Verification items for the finished model (mm, model axes). Face numbers are marked on the shaded views. A direction names the side the tool comes from. Round coordinates to 2 decimals unless told otherwise and drop trailing zeros. Write each loop counter-clockwise with the first axis right and the second up, starting at its lowest first coordinate (ties: lowest second). Pieces come first, ordered by that corner, then holes. Notation, with made-up numbers: (9, 36) - (40, 36) arc R30 ccw to (40, 65) - close; hole circle Ø3 at (-1.75, 30). An arc over 180 degrees is marked (long way). Answer as a JSON object with one key per item and string values. Group by question number.
1) Thickness scan on line 1 (X direction, y = 4, z = -8); line 2 (X direction, y = 5.5, z = -4); line 3 (X direction, y = 3.75, z = -3.25). Record the ranges inside material, lowest first.
2) Section check B-B (z = 0). Enter the section's corners in (x, y).
3) Set-up check for the marked faces 1, 2 and 3: record each of +Z, -Z, +X, -X, +Y, -Y from which the full face is reachable in a straight line by a thin tool's end or side.
4) Mould release check, pull along X, two halves, no side actions. Record for the marked faces 4, 5 and 6: +X half, -X half, draft (parallel to the pull), parting line (faces both ways), or undercut.
5) Section check D-D (x = 21). Enter the section's corners in (y, z).
6) Go/stop test with flat-tipped pins: pin 1 Ø1.5 at (x, y) = (14, 2) entering from -Z; pin 2 Ø3 at (x, y) = (10, 8) entering from -Z; pin 3 Ø2 at (x, z) = (18, -7) entering from +Y; pin 4 Ø2 at (x, z) = (27.5, -5.5) entering from +Y. Record where each tip stops, or that it passes through.
7) Section check A-A (y = 8). Enter the section's corners in (x, z), then the cut area to 3 significant figures.
```python
from build123d import *

# Parameters (mm, degrees)
F0_R     = 10
F1_DEPTH = 5
F2_R     = 7.5
F3_DEPTH = 5
F4_R     = 10
F5_DEPTH = 5
F6_R     = 5
F7_DEPTH = 20
F8_SIZE  = 1


with BuildPart() as f1:
    # F0 (on Right) → F1 (new body)
    with BuildSketch(Plane.YZ):
        Circle(F0_R)
    extrude(amount=F1_DEPTH)

    # F2 (on face) → F3 (join)
    with BuildSketch(Plane.YZ.offset(5)):
        Circle(F2_R)
    extrude(amount=F3_DEPTH)

    # F4 (on face) → F5 (join)
    with BuildSketch(Plane.YZ.offset(10)):
        Circle(F4_R)
    extrude(amount=F5_DEPTH)

    # F6 (on face) → F7 (join)
    with BuildSketch(Plane.YZ.offset(15)):
        Circle(F6_R)
    extrude(amount=F7_DEPTH)

    # F8
    f8_edges = [f1.edges().sort_by_distance(p)[0] for p in [
        (35, -5, 0),
    ]]
    chamfer(f8_edges, length=F8_SIZE)


solid = f1.part
```
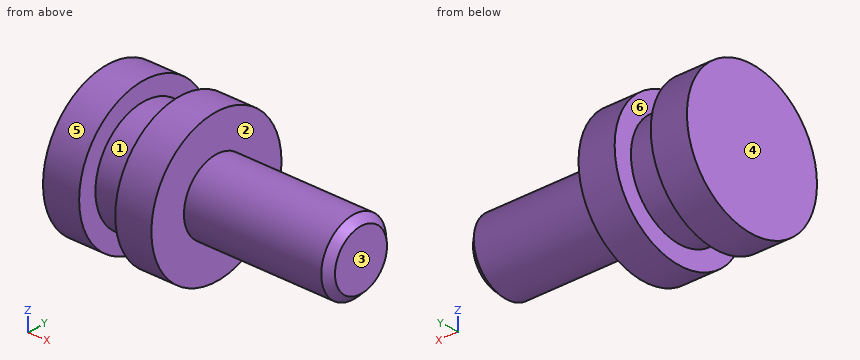
Returned:
{
 "1": {"line 1": "0 to 5, 10 to 15", "line 2": "0 to 15", "line 3": "0 to 34.04"},
 "2": {"outline": "(0, -10) - (5, -10) - (5, -7.5) - (10, -7.5) - (10, -10) - (15, -10) - (15, -5) - (34, -5) - (35, -4) - (35, 4) - (34, 5) - (15, 5) - (15, 10) - (10, 10) - (10, 7.5) - (5, 7.5) - (5, 10) - (0, 10) - close"},
 "3": {"face 1": "none", "face 2": "+X", "face 3": "+Z, -Z, +X, +Y, -Y"},
 "4": {"face 4": "-X half", "face 5": "draft", "face 6": "undercut"},
 "5": {"outline": "circle Ø10 at (0, 0)"},
 "6": {"pin 1": "z = -9.92", "pin 2": "z = -7.6", "pin 3": "through", "pin 4": "y = 2.18"},
 "7": {"outline": "(0, -6) - (5, -6) - (5, 6) - (0, 6) - close; (10, -6) - (15, -6) - (15, 6) - (10, 6) - close", "area": "120 mm2"}
}
